Build history of the part. All positions in model axes, mm. A direction names the side the tool comes from. Round coordinates to 2 decimals unless told otherwise and drop trailing zeros. Order: outer loops, then holes, each group sorted by start corner. A loop starts at its lowest first (then second) coordinate and runs counter-clockwise, first axis right, second up. Notation, with made-up numbers: M 40.5,-24.5 L 93.5,-24.5 A35 cw 93.5,12.5 Z; hole C 57,-36.5 d5. An arc over 180 degrees is marked long. Use CSV: the item, a comma, the result in double quotes.
from build123d import *

# Parameters (mm, degrees)
BOSS_EXTRUDE1_DEPTH = 24
SKETCH4_R           = 3.5
BOSS_EXTRUDE2_DEPTH = 6
SKETCH5_R           = 3.1
BOSS_EXTRUDE3_DEPTH = 6
DIAMETERHOLE1_D     = 3
DIAMETERHOLE1_DEPTH = 3
DIAMETERHOLE1_TIP   = 0.901290929
CUT_EXTRUDE1_DEPTH  = 3
DIAMETERHOLE3_D     = 9


with BuildPart() as part:
    # Sketch1 → Boss-Extrude1 (new body)
    with BuildSketch(Plane(origin=(0, 0, 0), x_dir=(0, 0, -1), z_dir=(1, 0, 0))):
        Polygon((-18, 42.5), (-18, 24), (-34.5, 24), (-35, 23.5), (-35, 0), (35, 0), (35, 23.5), (34.5, 24), (18, 24), (18, 42.5), (17.5, 43), (-17.5, 43), align=None)
    extrude(amount=BOSS_EXTRUDE1_DEPTH)

    # Sketch4 → Boss-Extrude2 (add)
    with BuildSketch(Plane(origin=(24, 0, 0), x_dir=(0, 0, -1), z_dir=(1, 0, 0))):
        Polygon((-17.75, 40.75), (-15.75, 42.75), (15.75, 42.75), (17.75, 40.75), (17.75, 9.25), (15.75, 7.25), (-15.75, 7.25), (-17.75, 9.25), align=None)
        with Locations((-13.05, 38.05)):
            Circle(SKETCH4_R, mode=Mode.SUBTRACT)
        with Locations((13.05, 38.05)):
            Circle(SKETCH4_R, mode=Mode.SUBTRACT)
        with Locations((-13.05, 11.95)):
            Circle(SKETCH4_R, mode=Mode.SUBTRACT)
        with Locations((13.05, 11.95)):
            Circle(SKETCH4_R, mode=Mode.SUBTRACT)
    extrude(amount=BOSS_EXTRUDE2_DEPTH)

    # Sketch5 → Boss-Extrude3 (add)
    with BuildSketch(Plane(origin=(24, 0, 0), x_dir=(0, 0, -1), z_dir=(1, 0, 0))):
        with Locations((-13.05, 38.05)):
            Circle(SKETCH5_R)
        with Locations((13.05, 38.05)):
            Circle(SKETCH5_R)
        with Locations((13.05, 11.95)):
            Circle(SKETCH5_R)
        with Locations((-13.05, 11.95)):
            Circle(SKETCH5_R)
    extrude(amount=BOSS_EXTRUDE3_DEPTH)

    # DiameterHole1
    with Locations(Plane(origin=(30, 0, 0), x_dir=(0, 0, -1), z_dir=(1, 0, 0))):
        with Locations((-13.05, 38.05), (13.05, 38.05), (-13.05, 11.95), (13.05, 11.95)):
            Hole(DIAMETERHOLE1_D / 2, depth=DIAMETERHOLE1_DEPTH)
            with Locations((0, 0, -(DIAMETERHOLE1_DEPTH + DIAMETERHOLE1_TIP / 2))):  # 118° drill point
                Cone(0, DIAMETERHOLE1_D / 2, DIAMETERHOLE1_TIP, mode=Mode.SUBTRACT)

    # Sketch8 → Cut-Extrude1 (cut)
    with BuildSketch(Plane(origin=(30, 0, 0), x_dir=(0, 0, -1), z_dir=(1, 0, 0))):
        Polygon((-13.05, 36.317949192), (-11.55, 37.183974596), (-11.55, 38.916025404), (-13.05, 39.782050808), (-14.55, 38.916025404), (-14.55, 37.183974596), align=None)
        Polygon((14.55, 37.183974596), (14.55, 38.916025404), (13.05, 39.782050808), (11.55, 38.916025404), (11.55, 37.183974596), (13.05, 36.317949192), align=None)
        Polygon((-11.55, 11.083974596), (-11.55, 12.816025404), (-13.05, 13.682050808), (-14.55, 12.816025404), (-14.55, 11.083974596), (-13.05, 10.217949192), align=None)
        Polygon((14.55, 11.083974596), (14.55, 12.816025404), (13.05, 13.682050808), (11.55, 12.816025404), (11.55, 11.083974596), (13.05, 10.217949192), align=None)
    extrude(amount=-CUT_EXTRUDE1_DEPTH, mode=Mode.SUBTRACT)

    # Sketch9 → Cut-Revolve1 (revolve, cut)
    with BuildSketch(Plane.XY, mode=Mode.PRIVATE) as cut_revolve1_sk:
        Polygon((0, 35.5), (3, 35.5), (3, 31), (6, 31), (6, 30), (22, 30), (22, 31), (24, 31), (24, 35.5), (30, 35.5), (30, 25), (0, 25), align=None)
    revolve(cut_revolve1_sk.sketch.rotate(Axis((30, 25, 0), (-1, 0, 0)), 90), axis=Axis((30, 25, 0), (-1, 0, 0)), mode=Mode.SUBTRACT)

    # DiameterHole3 (through all)
    with Locations(Plane(origin=(0, 24, 0), x_dir=(1, 0, 0), z_dir=(0, 1, 0))):
        with Locations((12, -26), (12, 26)):
            Hole(DIAMETERHOLE3_D / 2)


solid = part.part
(1) Tool access for faces 1 (the face through (28.521, 13.243, -13.811)), 2 (the face through (1.521, 16.146, -5.645)), 3 (the face through (14.11, 29.88, 1.08)): list every direction of +Z, -Z, +X, -X, +Y, -Y with a clear straight run to the whole face (end or side of a thin tool).
Answer block:
face 1,"+X"
face 2,"-X"
face 3,"+X, -X"
(2) Cut at C-C, the plane y = 17. Give the cut face in (x, z), and give its area (3 significant figures).
Answer block:
outline,"M 0,-35 L 24,-35 L 24,-17.75 L 30,-17.75 L 30,-6.8 L 24,-6.8 L 24,6.8 L 30,6.8 L 30,17.75 L 24,17.75 L 24,35 L 0,35 L 0,6.8 L 3,6.8 L 3,-6.8 L 0,-6.8 Z; hole C 12,-26 d9; hole C 12,26 d9"
area,"1,640 mm²"
(3) Drop flat-ended pins along their axis: pin 1 (0.9 mm diameter, centred on x = 29, y = 38, fed in from +Z); pin 2 (13 mm diameter, centred on x = 17, z = 26, fed in from +Y); pin 3 (0.8 mm diameter, centred on y = 37.5, z = 12, fed in from +X); pin 4 (1.5 mm diameter, centred on x = 11, z = -22.5, fed in from -Y). Give the stop position or say it passes through.
Answer block:
pin 1,"stops at z = 17.75"
pin 2,"stops at y = 24"
pin 3,"stops at x = 27"
pin 4,"passes through"
(4) Cut at B-B, the plane x = 14.5. Give the cut face in (y, z), and give its area (3 significant figures).
Answer block:
outline,"M 0,-35 L 23.5,-35 L 24,-34.5 L 24,-29.74 L 0,-29.74 Z; M 0,-22.26 L 24,-22.26 L 24,-18 L 42.5,-18 L 43,-17.5 L 43,17.5 L 42.5,18 L 24,18 L 24,22.26 L 0,22.26 Z; M 0,29.74 L 24,29.74 L 24,34.5 L 23.5,35 L 0,35 Z; hole C 25,0 d10"
area,"1,930 mm²"
(5) Two-plate mould, pull along Y, no slides. Class faces 4 (the face through (29, 12, 14.55)), 5 (the face through (27, 41.7, 16.8)), 6 (the face through (30, 10.6, 11.7)): released by +Y, released by -Y, zero draft, split by the parting line, or undercut.
Answer block:
face 4,"undercut"
face 5,"released by +Y"
face 6,"zero draft"
(6) Cut at D-D, the plane z = 26. Give the cut face in (x, y).
Answer block:
outline,"M 0,0 L 7.5,0 L 7.5,24 L 0,24 Z; M 16.5,0 L 24,0 L 24,24 L 16.5,24 Z"
(7) Cut at A-A, the plane z = 0. Give the cut face in (x, y), and give its area (3 significant figures).
Answer block:
outline,"M 0,0 L 24,0 L 24,7.25 L 30,7.25 L 30,14.5 L 24,14.5 L 24,19 L 22,19 L 22,20 L 6,20 L 6,19 L 3,19 L 3,14.5 L 0,14.5 Z; M 0,35.5 L 3,35.5 L 3,31 L 6,31 L 6,30 L 22,30 L 22,31 L 24,31 L 24,35.5 L 30,35.5 L 30,42.75 L 24,42.75 L 24,43 L 0,43 Z"
area,"836 mm²"
(8) Wall check: line 1 (Z direction, x = 12, y = 7); line 2 (Z direction, x = 1.4, y = 25); line 3 (Y direction, x = 5.2, z = 0). Give the ranges that are in metal, low to high. Write a range as from..to.
Answer block:
line 1,"z = -35..-30.5, -21.5..21.5, 30.5..35"
line 2,"z = -18..-10.5, 10.5..18"
line 3,"y = 0..19, 31..43"
